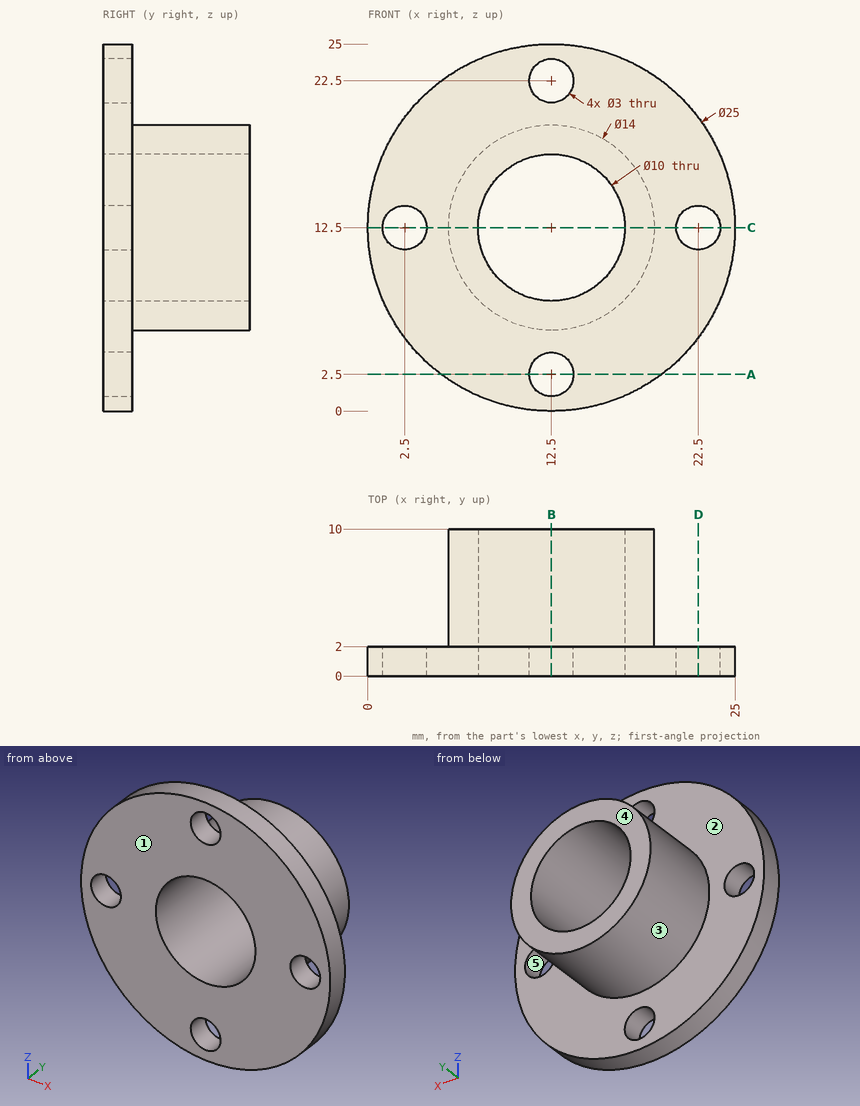
Could you check a few things on this drawing? It's one solid part, dimensions in mm from its lowest x, y, z. A direction names the side the tool comes from. Round coordinates to 2 decimals unless told otherwise and drop trailing zeros. Write each loop counter-clockwise with the first axis right and the second up, starting at its lowest first coordinate (ties: lowest second). Pieces come first, ordered by that corner, then holes. Notation, with made-up numbers: (86.5, 45) -> (126.5, 45) arc R17 cw to (126.5, 52) -> close; hole circle Ø5 at (-8, -18.75). An arc over 180 degrees is marked (long way). One line per question, with ' | ' between items. Start each with the question number.
1) Suppose I cut it at D-D on x = 22.5. Write out the boundary of the cut face in (y, z).
2) Suppose I cut it at A-A on z = 2.5. Write out the boundary of the cut face in (x, y).
3) I need wall thicknesses on line 1 (Y direction, x = 7.25, z = 17.25); line 2 (Z direction, x = 12.5, y = 5.5); line 3 (X direction, y = 7.5, z = 12). Which ranges of each line are inside material? Lowest first, please. Write a range as [from, to].
4) If we mould it in two halves opening along Z, with no side actions, what happens to the marked faces 3, 4 and 5? For each: released by +Z, released by -Z, zero draft, split by the parting line, or undercut.
5) Suppose I cut it at C-C on z = 12.5. Write out the boundary of the cut face in (x, y), then the cut area to 3 significant figures.
6) I'm going to push flat-ended pins straight in: P1, Ø3, axis at y = 5, z = 19.5, coming from the -X side; P2, Ø4, axis at x = 12.5, z = 22.5, coming from the +Y side; P3, Ø4, axis at x = 19, z = 18.5, coming from the +Y side; P4, Ø4, axis at y = 8, z = 10.5, coming from the -X side. Where does each tip first touch, or does it pass through?
7) Suppose I cut it at B-B on x = 12.5. Write out the boundary of the cut face in (y, z), then the cut area to 3 significant figures.
8) On a 3-axis mill with a long thin cutter (end or side, diameter ignored), from which of +Z, -Z, +X, -X, +Y, -Y can I reach the whole of each face in a straight line? I mean the marked faces 1 and 2. Say none if no direction works.
Return value:
1) outline: (0, 5) -> (2, 5) -> (2, 11) -> (0, 11) -> close; (0, 14) -> (2, 14) -> (2, 20) -> (0, 20) -> close
2) outline: (5, 0) -> (11, 0) -> (11, 2) -> (5, 2) -> close; (14, 0) -> (20, 0) -> (20, 2) -> (14, 2) -> close
3) line 1: y = [0, 2] | line 2: z = [5.5, 7.5], [17.5, 19.5] | line 3: x = [5.52, 7.53], [17.47, 19.48]
4) face 3: split by the parting line | face 4: zero draft | face 5: undercut
5) outline: (0, 0) -> (1, 0) -> (1, 2) -> (0, 2) -> close; (4, 0) -> (7.5, 0) -> (7.5, 10) -> (5.5, 10) -> (5.5, 2) -> (4, 2) -> close; (17.5, 0) -> (21, 0) -> (21, 2) -> (19.5, 2) -> (19.5, 10) -> (17.5, 10) -> close; (24, 0) -> (25, 0) -> (25, 2) -> (24, 2) -> close | area: 50.0 mm2
6) P1: stops at x = 8.17 | P2: stops at y = 2 | P3: stops at y = 10 | P4: stops at x = 5.5
7) outline: (0, 0) -> (2, 0) -> (2, 1) -> (0, 1) -> close; (0, 4) -> (2, 4) -> (2, 5.5) -> (10, 5.5) -> (10, 7.5) -> (0, 7.5) -> close; (0, 17.5) -> (10, 17.5) -> (10, 19.5) -> (2, 19.5) -> (2, 21) -> (0, 21) -> close; (0, 24) -> (2, 24) -> (2, 25) -> (0, 25) -> close | area: 50.0 mm2
8) face 1: +Z, -Z, +X, -X, -Y | face 2: +Y
